Could you check a few things on this drawing? It's one solid part, dimensions in mm from its lowest x, y, z. A direction names the side the tool comes from. Give positions to 0.01 mm unless a question says otherwise; leave off trailing zeros. Order: outer loops, then holes, each group sorted by start corner. A loop starts at its lowest first (then second) coordinate and runs counter-clockwise, first axis right, second up.
Item 1: I want a section at D-D, the plane x = 27. Write out the boundary of the cut face in (y, z).
Item 2: I want a section at A-A, the plane x = 4. Write out the boundary of the cut face in (y, z), then the cut area to 3 significant figures.
Item 3: If we mould it in two halves opening along X, with no side actions, what happens to the marked faces 3, 4 and 5? For each: +X half, -X half, draft (parallel to the pull), parting line (faces both ways), or undercut.
Item 4: Which directions (+Z, -Z, +X, -X, +Y, -Y) give clear straight access to the entire face, cutting with the end or side of a thin tool? Please do the marked faces 1 and 2.
Item 5: If I drill on line 1 along X through (y, z) = (17.65, 29.3); line 2 along X through (y, z) = (17.65, 29.15); line 3 along Y through (x, z) = (27, 28), over which ranges is the centre line in solid material (lowest first)?
Item 6: I'm going to push flat-ended pins straight in: pin 1 Ø1 at (y, z) = (23, 13.5) entering from -X; pin 2 Ø9 at (x, y) = (42, 11.5) entering from -Z; pin 3 Ø8 at (x, y) = (12.5, 5.5) entering from -Z. Where does each tip first touch, or does it pass through?
Item 7: I want a section at B-B, the plane z = 26. Write out the boundary of the cut face in (x, y), then the cut area to 3 significant figures.
Item 8: I want a section at C-C, the plane y = 17.65. Count the separate pieces of the cut face and the enclosed holes in it, then the cut area to 3 significant figures.
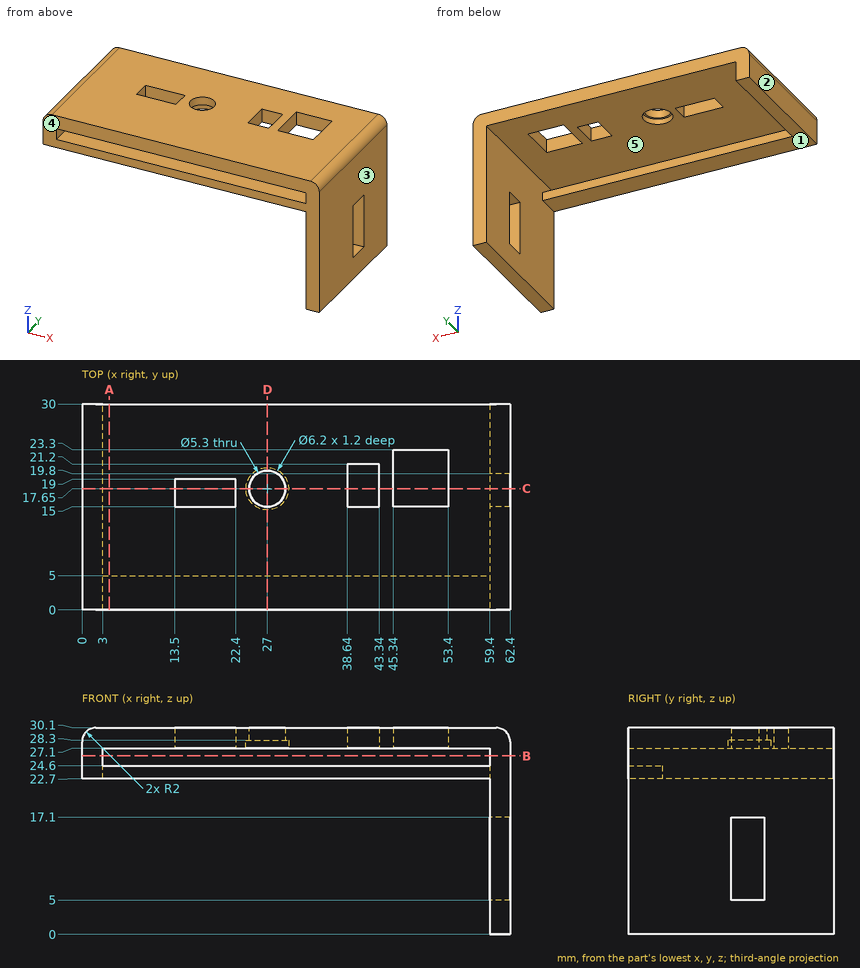
Results list:
1. outline: (0, 22.7) - (5, 22.7) - (5, 24.6) - (0, 24.6) - close; (0, 27.1) - (14.55, 27.1) - (14.55, 28.3) - (15, 28.3) - (15, 30.1) - (0, 30.1) - close; (20.3, 28.3) - (20.75, 28.3) - (20.75, 27.1) - (30, 27.1) - (30, 30.1) - (20.3, 30.1) - close
2. outline: (0, 22.7) - (5, 22.7) - (5, 24.6) - (0, 24.6) - close; (0, 27.1) - (30, 27.1) - (30, 30.1) - (0, 30.1) - close
2. area: 99.5 mm2
3. face 3: +X half
3. face 4: draft
3. face 5: undercut
4. face 1: -Z, -X, +Y, -Y
4. face 2: +Z, -Z, -X, +Y, -Y
5. line 1: x = 0.4 to 13.5, 22.4 to 24.35, 29.65 to 38.64, 43.34 to 45.34, 53.4 to 62
5. line 2: x = 0.3 to 13.5, 22.4 to 24.35, 29.65 to 38.64, 43.34 to 45.34, 53.4 to 62.1
5. line 3: y = 0 to 14.55, 20.75 to 30
6. pin 1: stops at x = 59.4
6. pin 2: stops at z = 27.1
6. pin 3: stops at z = 22.7
7. outline: (0, 0) - (3, 0) - (3, 30) - (0, 30) - close; (59.4, 0) - (62.4, 0) - (62.4, 30) - (59.4, 30) - close
7. area: 180 mm2
8. separate pieces: 6
8. enclosed holes: 0
8. area: 162 mm2
